Solid Edge part; units mm, degrees
sketch "Sketch1" plane through (0, 0, 0) normal (0, 0, 1) x (1, 0, 0)
  line L0 (2.0207, -3.5) -> (-2.0207, -3.5)
  line L1 (-4.0415, 0) -> (-2.0207, -3.5)
  line L2 (-2.0207, 3.5) -> (-4.0415, 0)
  line L3 (-2.0207, 3.5) -> (2.0207, 3.5)
  line L4 (2.0207, 3.5) -> (4.0415, 0)
  line L5 (4.0415, 0) -> (2.0207, -3.5)
extrude "Protrusion1" add sketch "Sketch1" along normal mid plane 3.1
hole "Hole_1" at (0, 0, 1.55) direction (0, 0, -1) diameter 3.242 end through all
sketch "Sketch2" plane through (0, 0, 0) normal (1, 0, 0) x (0, 1, 0)
  line L0 (-3.5, 1.55) -> (-1.7885, 3.2615)
revolve "RevolvedCutout1" cut sketch "Sketch2" angle 360 about axis through (0, 0, -57) along (0, 0, 1) material side at (0, -2.6796, 2.4411)
mirror "Mirror1" about plane through (0, 0, 0) normal (0, 0, 1) of "RevolvedCutout1"
Build history of the part. All positions in model axes, mm. Give positions to 0.01 mm unless a question says otherwise; leave off trailing zeros. Loops run counter-clockwise (first coordinate to the right, second up) from the corner with the lowest first, then second, coordinate; pieces in that order, holes last. Notation, with made-up numbers: (71, 43) -> (82, 43) arc R17 ccw to (82, 64) -> close; hole circle Ø8 at (-1.5, 29.25). An arc over 180 degrees is marked (long way). One line per question, with ' | ' between items. Start each with the question number.
1) Probe L1, parallel to Y at x = 0, z = 0.3; L2, parallel to Y at x = -1.25, z = -0.3; L3, parallel to X at y = -1.25, z = -1.3. List the from-to ranges inside material, lowest first.
2) Cut at A-A (z = 0.5). Give the cut face in (x, y), plus the area to 3 significant figures.
3) Pin check, flat tip, straight feed: pin 1 (3 mm diameter, centred on x = 0, y = 0, fed in from -Z). Stop position of the tip, or through.
4) Two-plate mould, pull along X, no slides. Class faces 1 (the flat face through (-3, 1.8, 0)), 2 (the cylindrical face through (-1.438, -0.748, 0.022)), 3 (the flat face through (0, 3.5, 0)): released by +X, released by -X, zero draft, split by the parting line, or undercut.
Return value:
1) L1: -3.5 to -1.62, 1.62 to 3.5 | L2: -3.5 to -1.03, 1.03 to 3.5 | L3: -3.32 to -1.03, 1.03 to 3.32
2) outline: (-4.04, 0) -> (-2.02, -3.5) -> (2.02, -3.5) -> (4.04, 0) -> (2.02, 3.5) -> (-2.02, 3.5) -> close; hole circle Ø3.24 at (0, 0) | area: 34.2 mm^2
3) pin 1: through
4) face 1: released by -X | face 2: undercut | face 3: zero draft
